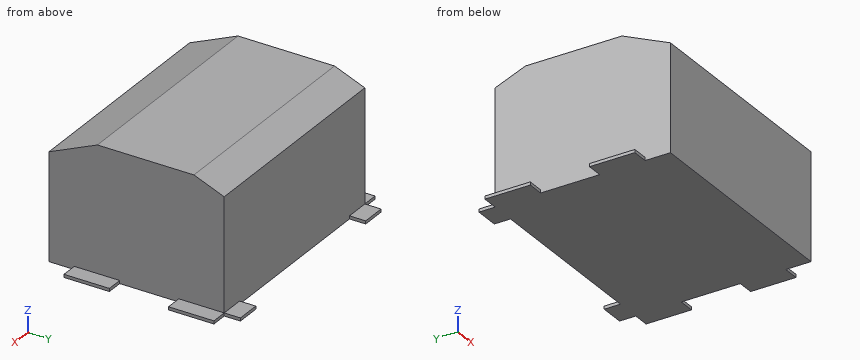
from build123d import *

# Parameters (mm, degrees)
SKETCH1_W           = 465.838
SKETCH1_H           = 367.518
BOSS_EXTRUDE1_DEPTH = 3.175
SKETCH2_W           = 3.175
SKETCH2_H           = 308.082
SKETCH2_W_2         = 87.632
SKETCH2_W_3         = 89.789
SKETCH2_W_4         = 459.488
SKETCH2_H_2         = 50.8
BOSS_EXTRUDE2_DEPTH = 200.6
SKETCH11_W          = 87.632
SKETCH11_H          = 308.082
SKETCH11_W_2        = 89.789
SKETCH11_W_3        = 3.175
SKETCH11_W_4        = 459.488
SKETCH11_H_2        = 50.8
SKETCH11_H_3        = 3.175
BOSS_EXTRUDE8_DEPTH = 64.05
SKETCH10_W          = 34.036
SKETCH10_H          = 95.25
SKETCH10_W_2        = 50.8
SKETCH10_H_2        = 34.036
BOSS_EXTRUDE7_DEPTH = 6.35
CUT_EXTRUDE1_DEPTH  = 605.839795074


with BuildPart() as part:
    # Sketch1 → Boss-Extrude1 (new body)
    with BuildSketch(Plane.XY):
        with Locations((-46.4825, -26.543)):
            Rectangle(SKETCH1_W, SKETCH1_H)
    extrude(amount=BOSS_EXTRUDE1_DEPTH)

    # Sketch2 → Boss-Extrude2 (add)
    with BuildSketch(Plane.XY.offset(3.175)):
        Polygon((186.4365, -210.302), (186.4365, -157.216), (183.2615, -157.216), (183.2615, -208.016), (-276.2265, -208.016), (-276.2265, -157.216), (-279.4015, -157.216), (-279.4015, -210.302), align=None)
        Polygon((183.2615, 154.041), (186.4365, 154.041), (186.4365, 157.216), (-279.4015, 157.216), (-279.4015, -157.216), (-276.2265, -157.216), (183.2615, -157.216), (186.4365, -157.216), (186.4365, -154.041), (183.2615, -154.041), (93.4725, -154.041), (90.2975, -154.041), (0.5085, -154.041), (-2.6665, -154.041), (-92.4555, -154.041), (-95.6305, -154.041), (-185.4195, -154.041), (-188.5945, -154.041), (-276.2265, -154.041), (-276.2265, 154.041), (-188.5945, 154.041), (-185.4195, 154.041), (-95.6305, 154.041), (-92.4555, 154.041), (-2.6665, 154.041), (0.5085, 154.041), (90.2975, 154.041), (93.4725, 154.041), align=None)
        with Locations((184.849, 0)):
            Rectangle(SKETCH2_W, SKETCH2_H)
        with Locations((91.885, 0)):
            Rectangle(SKETCH2_W, SKETCH2_H)
        with Locations((-187.007, 0)):
            Rectangle(SKETCH2_W, SKETCH2_H)
        with Locations((-94.043, 0)):
            Rectangle(SKETCH2_W, SKETCH2_H)
        with Locations((-1.079, 0)):
            Rectangle(SKETCH2_W, SKETCH2_H)
        with Locations((-232.4105, 0)):
            Rectangle(SKETCH2_W_2, SKETCH2_H)
        with Locations((-140.525, 0)):
            Rectangle(SKETCH2_W_3, SKETCH2_H)
        with Locations((-47.561, 0)):
            Rectangle(SKETCH2_W_3, SKETCH2_H)
        with Locations((45.403, 0)):
            Rectangle(SKETCH2_W_3, SKETCH2_H)
        with Locations((138.367, 0)):
            Rectangle(SKETCH2_W_3, SKETCH2_H)
        with Locations((-46.4825, -182.616)):
            Rectangle(SKETCH2_W_4, SKETCH2_H_2)
    extrude(amount=BOSS_EXTRUDE2_DEPTH)

    # Sketch11 → Boss-Extrude8 (add)
    with BuildSketch(Plane.XY.offset(203.775)):
        with Locations((-232.4105, 0)):
            Rectangle(SKETCH11_W, SKETCH11_H)
        with Locations((-140.525, 0)):
            Rectangle(SKETCH11_W_2, SKETCH11_H)
        with Locations((-187.007, 0)):
            Rectangle(SKETCH11_W_3, SKETCH11_H)
        Polygon((-276.2265, -157.216), (183.2615, -157.216), (183.2615, -154.041), (93.4725, -154.041), (90.2975, -154.041), (0.5085, -154.041), (-2.6665, -154.041), (-92.4555, -154.041), (-95.6305, -154.041), (-185.4195, -154.041), (-188.5945, -154.041), (-276.2265, -154.041), align=None)
        with Locations((-46.4825, -182.616)):
            Rectangle(SKETCH11_W_4, SKETCH11_H_2)
        with Locations((-47.561, 0)):
            Rectangle(SKETCH11_W_2, SKETCH11_H)
        with Locations((-94.043, 0)):
            Rectangle(SKETCH11_W_3, SKETCH11_H)
        with Locations((45.403, 0)):
            Rectangle(SKETCH11_W_2, SKETCH11_H)
        with Locations((-1.079, 0)):
            Rectangle(SKETCH11_W_3, SKETCH11_H)
        with Locations((138.367, 0)):
            Rectangle(SKETCH11_W_2, SKETCH11_H)
        with Locations((91.885, 0)):
            Rectangle(SKETCH11_W_3, SKETCH11_H)
        with Locations((184.849, 0)):
            Rectangle(SKETCH11_W_3, SKETCH11_H)
        with Locations((184.849, -155.6285)):
            Rectangle(SKETCH11_W_3, SKETCH11_H_3)
        Polygon((-279.4015, -210.302), (186.4365, -210.302), (186.4365, -157.216), (183.2615, -157.216), (183.2615, -208.016), (-276.2265, -208.016), (-276.2265, -157.216), (-279.4015, -157.216), align=None)
        Polygon((-279.4015, 157.216), (-279.4015, -157.216), (-276.2265, -157.216), (-276.2265, -154.041), (-276.2265, 154.041), (-188.5945, 154.041), (-185.4195, 154.041), (-95.6305, 154.041), (-92.4555, 154.041), (-2.6665, 154.041), (0.5085, 154.041), (90.2975, 154.041), (93.4725, 154.041), (183.2615, 154.041), (186.4365, 154.041), (186.4365, 157.216), align=None)
    extrude(amount=BOSS_EXTRUDE8_DEPTH)

    # Sketch10 → Boss-Extrude7 (add)
    with BuildSketch(Plane.XY):
        with Locations((203.4545, 109.591)):
            Rectangle(SKETCH10_W, SKETCH10_H)
        with Locations((203.4545, -109.591)):
            Rectangle(SKETCH10_W, SKETCH10_H)
        with Locations((161.0365, 174.234)):
            Rectangle(SKETCH10_W_2, SKETCH10_H_2)
    boss_extrude7 = extrude(amount=BOSS_EXTRUDE7_DEPTH)

    # Mirror1: Boss-Extrude7 across plane
    add(boss_extrude7.mirror(Plane.ZY.offset(46.4825)))

    # Sketch12 → Cut-Extrude1 (cut, through all)
    with BuildSketch(Plane(origin=(186.4365, 0, 0), x_dir=(0, 0, -1), z_dir=(1, 0, 0))):
        Polygon((-267.825, -210.302), (-223.375, -210.302), (-267.825, -108.702), align=None)
        Polygon((-267.825, 157.216), (-267.825, 93.716), (-242.425, 157.216), align=None)
    extrude(amount=-CUT_EXTRUDE1_DEPTH, mode=Mode.SUBTRACT)


solid = part.part
Read the model definition and answer for the solid it produces. Units are mm, in the model's axes. Coordinates: 2 decimals unless noted, no trailing zeros. Loops run counter-clockwise (first coordinate to the right, second up) from the corner with the lowest first, then second, coordinate; pieces in that order, holes last.
Q1. The part is cut by section C-C on z = 154. Write down the section's boundary in (x, y), and give its area (3 significant figures).
Q2. Consider probe 1 along Y at (x, z) = (-11.5, 40); probe 2 along X at (y, z) = (25.5, 193.5); probe 3 along Z at (x, y) = (-143.5, 94). Determine where each line is inside the solid, lowest interval first.
Q3. The part is cut by section A-A on x = -132. Write down the section's boundary in (y, z) (3 decimals).
Q4. Each of these flat-tipped pins is pushed along its axis until it touches: pin 1 Ø5 at (y, z) = (-59.5, 127) entering from -X; pin 2 Ø17 at (x, y) = (-289.5, 117.5) entering from +Z; pin 3 Ø5 at (x, y) = (-197.5, -98) entering from -Z; pin 4 Ø1.9 at (x, z) = (-290.5, 4.5) entering from -Y. Where does it stop, or does it pass through?
Q5. The part is cut by section B-B on y = -137. Write down the section's boundary in (x, z), and give its area (3 significant figures).
Q6. The part is cut by section D-D on y = 29. Write down the section's boundary in (x, z) (1 decimal).
Results below:
1. outline: (-279.4, -210.3) - (186.44, -210.3) - (186.44, 157.22) - (-279.4, 157.22) - close
1. area: 171,000 mm2
2. probe 1: y = -210.3 to 157.22
2. probe 2: x = -279.4 to 186.44
2. probe 3: z = 0 to 267.71
3. outline: (-210.302, 0) - (157.216, 0) - (157.216, 242.425) - (93.716, 267.825) - (-108.702, 267.825) - (-210.302, 223.375) - close
4. pin 1: stops at x = -279.4
4. pin 2: stops at z = 6.35
4. pin 3: stops at z = 0
4. pin 4: stops at y = -157.22
5. outline: (-313.44, 0) - (220.47, 0) - (220.47, 6.35) - (186.44, 6.35) - (186.44, 255.44) - (-279.4, 255.44) - (-279.4, 6.35) - (-313.44, 6.35) - close
5. area: 119,000 mm2
6. outline: (-279.4, 0) - (186.4, 0) - (186.4, 267.8) - (-279.4, 267.8) - close
